from build123d import *

# Parameters (mm, degrees)
BOSS_EXTRU_1_DEPTH                                 = 15
CHAMBRAGE_POUR_VIS_T_TE_HEXAGONALE_M51_D           = 5.5
CHAMBRAGE_POUR_VIS_T_TE_HEXAGONALE_M51_CBORE_D     = 10
CHAMBRAGE_POUR_VIS_T_TE_HEXAGONALE_M51_CBORE_DEPTH = 5.4


with BuildPart() as part:
    # Esquisse1 → Boss.-Extru.1 (new, symmetric)
    with BuildSketch(Plane.XY):
        with BuildLine():
            Line((43.383109312, -1.070799618), (67.609389379, -1.070799618))
            ThreePointArc((67.609389379, -1.070799618), (87.383109312, 15.929200382), (107.156829246, -1.070799618))
            Line((107.156829246, -1.070799618), (131.383109312, -1.070799618))
            Line((131.383109312, -1.070799618), (131.383109312, 13.929200382))
            Line((131.383109312, 13.929200382), (111.383109312, 13.929200382))
            ThreePointArc((111.383109312, 13.929200382), (87.383109312, 25.929200382), (63.383109312, 13.929200382))
            Line((63.383109312, 13.929200382), (43.383109312, 13.929200382))
            Line((43.383109312, 13.929200382), (43.383109312, -1.070799618))
        make_face()
    extrude(amount=BOSS_EXTRU_1_DEPTH, both=True)

    # Chambrage pour vis à tête hexagonale M51 (through all)
    with Locations(Plane(origin=(53.383109312, 13.929200382, 0), x_dir=(0, 0, 1), z_dir=(0, 1, 0))):
        with Locations((0, 0), (0, 68)):
            CounterBoreHole(CHAMBRAGE_POUR_VIS_T_TE_HEXAGONALE_M51_D / 2, CHAMBRAGE_POUR_VIS_T_TE_HEXAGONALE_M51_CBORE_D / 2, CHAMBRAGE_POUR_VIS_T_TE_HEXAGONALE_M51_CBORE_DEPTH)


solid = part.part
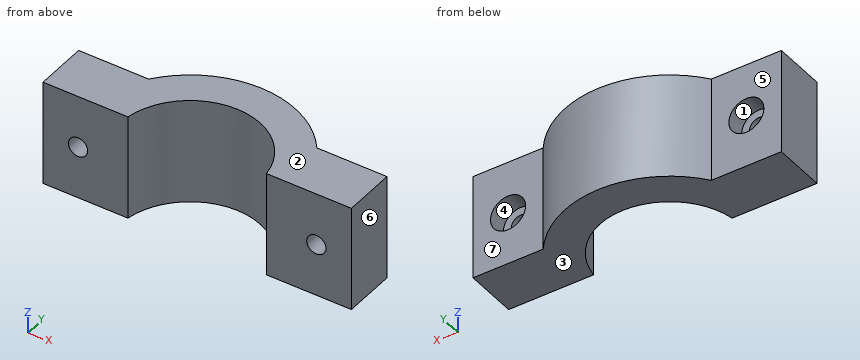
Model file for the job. Use its own axes, mm. Face numbers are marked on the shaded views. A direction names the side the tool comes from. Give positions to 0.01 mm unless a question says otherwise; leave off trailing zeros. Order: outer loops, then holes, each group sorted by start corner. A loop starts at its lowest first (then second) coordinate and runs counter-clockwise, first axis right, second up. Notation, with made-up numbers: (27.25, 61) - (79.25, 61) arc R19 ccw to (79.25, 68) - close; hole circle Ø8 at (-24.75, -30.5). An arc over 180 degrees is marked (long way). Write item = value, one per line. Start each with the question number.
1. Cut at D-D, the plane y = 19.5. List the corners of the cut face in (x, z).
2. Cut at B-B, the plane y = 2.25. List the corners of the cut face in (x, z).
3. Cut at C-C, the plane y = 5.75. List the corners of the cut face in (x, z), and give its area (3 significant figures).
4. Which spindle directions (+Z, -Z, +X, -X, +Y, -Y) get a long thin tool onto all of the face, cutting with end or side? Do the marked faces 4, 5, 6 and 7. Say none if no direction does.
5. Probe line 1 along X through (y, z) = (3.5, 0); line 2 along X through (y, z) = (3, 0); line 3 along Z through (x, y) = (122, 7.5). List the from-to ranges inside material, lowest first.
6. Cut at A-A, the plane z = 0. List the corners of the cut face in (x, y).
7. Drop flat-ended pins along their axis: P1, Ø4.5, axis at x = 53.38, z = 0, coming from the -Y side; P2, Ø16, axis at x = 125.5, z = 1.5, coming from the +Y side; P3, Ø3, axis at x = 78.5, z = 8.5, coming from the +Y side; P4, Ø6, axis at x = 53.38, z = 0, coming from the +Y side. Give the stop position or say it passes through.
8. Two-plate mould, pull along Z, no slides. Class the marked faces 1, 2 and 3: pulls with the +Z half, pulls with the -Z half, needs draft (parallel to the pull), parting line crosses it, or undercut.
Taken from the geometry:
q1.outline = (68.82, -15) - (105.94, -15) - (105.94, 15) - (68.82, 15) - close
q2.outline = (43.38, -15) - (68.41, -15) - (68.41, 15) - (43.38, 15) - close; (106.36, -15) - (131.38, -15) - (131.38, 15) - (106.36, 15) - close; hole circle Ø5.5 at (53.38, 0); hole circle Ø5.5 at (121.38, 0)
q3.outline = (43.38, -15) - (69.96, -15) - (69.96, 15) - (43.38, 15) - close; (104.81, -15) - (131.38, -15) - (131.38, 15) - (104.81, 15) - close; hole circle Ø5.5 at (53.38, 0); hole circle Ø5.5 at (121.38, 0)
q3.area = 1,550 mm²
q4.face_4 = +Y
q4.face_5 = +Z, -Z, -X, +Y
q4.face_6 = +Z, -Z, +X, +Y, -Y
q4.face_7 = +Z, -Z, +X, +Y
q5.line_1 = 43.38 to 50.63, 56.13 to 68.87, 105.89 to 118.63, 124.13 to 131.38
q5.line_2 = 43.38 to 50.63, 56.13 to 68.67, 106.09 to 118.63, 124.13 to 131.38
q5.line_3 = -15 to -2.68, 2.68 to 15
q6.outline = (43.38, -1.07) - (50.63, -1.07) - (50.63, 8.53) - (48.38, 8.53) - (48.38, 13.93) - (43.38, 13.93) - close; (56.13, -1.07) - (67.61, -1.07) arc R20 cw to (107.16, -1.07) - (118.63, -1.07) - (118.63, 8.53) - (116.38, 8.53) - (116.38, 13.93) - (111.38, 13.93) arc R30 ccw to (63.38, 13.93) - (58.38, 13.93) - (58.38, 8.53) - (56.13, 8.53) - close; (124.13, -1.07) - (131.38, -1.07) - (131.38, 13.93) - (126.38, 13.93) - (126.38, 8.53) - (124.13, 8.53) - close
q7.P1 = through
q7.P2 = 13.93
q7.P3 = 25.01
q7.P4 = 8.53
q8.face_1 = undercut
q8.face_2 = pulls with the +Z half
q8.face_3 = pulls with the -Z half
